from build123d import *

# Parameters (mm, degrees)
F0_W     = 10
F0_H     = 10
F1_DEPTH = 20
F2_DEPTH = 10
F3_R     = 0.5


with BuildPart() as f1:
    # F0 (on Front) → F1 (new body)
    with BuildSketch(Plane.XZ):
        with Locations((-5, 0)):
            Rectangle(F0_W, F0_H)
    extrude(amount=F1_DEPTH)

    # F0 (on Front) → F2 (join)
    with BuildSketch(Plane.XZ):
        with Locations((5, 0)):
            Rectangle(F0_W, F0_H)
        with Locations((-5, 0)):
            Rectangle(F0_W, F0_H)
    extrude(amount=F2_DEPTH)

    # F3
    f3_edges = [f1.edges().sort_by_distance(p)[0] for p in [
        (0, 0, 5),
        (10, -5, 5),
        (5, -10, 5),
        (0, -15, 5),
        (-5, -20, 5),
        (-10, -10, 5),
        (0, 0, -5),
        (-10, -10, -5),
        (-5, -20, -5),
        (0, -15, -5),
        (5, -10, -5),
        (10, -5, -5),
        (10, 0, 0),
        (-10, 0, 0),
        (0, -20, 0),
        (-10, -20, 0),
        (10, -10, 0),
    ]]
    fillet(f3_edges, radius=F3_R)


solid = f1.part
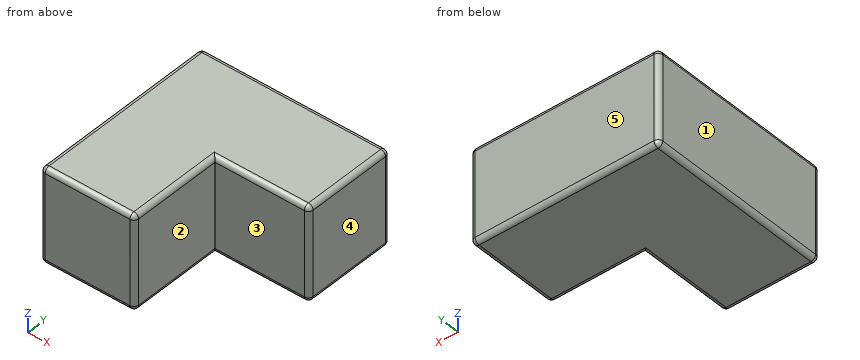
Source: CAD feature listing. Evaluate the final solid. Frame: model axes, mm. Face numbers are marked on the shaded views. A direction names the side the tool comes from. Coordinates: 2 decimals unless noted, no trailing zeros. Order: outer loops, then holes, each group sorted by start corner. A loop starts at its lowest first (then second) coordinate and runs counter-clockwise, first axis right, second up. Notation, with made-up numbers: M 11,25 L 26,25 A27 cw 26,45 Z; hole C 72,-5.75 d9. An arc over 180 degrees is marked long. Write each question's results on one line, items separated by ' | '. Start each with the question number.
Item 1: Cut plane A-A (x = 5.5). Return loops of the section in (y, z).
Item 2: Cut plane B-B (z = -2.5). Return loops of the section in (x, y).
Item 3: First-contact query: pin 1 Ø5 at (x, y) = (3, -14.5) entering from -Z; pin 2 Ø2.5 at (y, z) = (-16, 0) entering from +X; pin 3 Ø2.5 at (x, z) = (3, -1.5) entering from -Y. Flat tips, straight axial feed; report the tip coordinate or a pass-through.
Item 4: Draft query along Y for the marked faces 3, 4 and 5. Return one class per face: pulls with the +Y half, pulls with the -Y half, needs draft (parallel to the pull), parting line crosses it, or undercut.
Item 5: Set-up query: the marked faces 1 and 2. Return all of +Z, -Z, +X, -X, +Y, -Y with unobstructed straight access to the full face (end or side cutting, diameter ignored); none if empty.
Item 6: Line query: probe 1 along X at (y, z) = (-11.5, -0.25). Output: solid intervals per line, ascending.
Checked values:
1) outline: M -10,-4.5 A0.5 ccw -9.5,-5 L -0.5,-5 A0.5 ccw 0,-4.5 L 0,4.5 A0.5 ccw -0.5,5 L -9.5,5 A0.5 ccw -10,4.5 Z
2) outline: M -10,-19.5 A0.5 ccw -9.5,-20 L -0.5,-20 A0.5 ccw 0,-19.5 L 0,-10 L 9.5,-10 A0.5 ccw 10,-9.5 L 10,-0.5 A0.5 ccw 9.5,0 L -9.5,0 A0.5 ccw -10,-0.5 Z
3) pin 1: passes through | pin 2: stops at x = 0 | pin 3: stops at y = -10
4) face 3: pulls with the -Y half | face 4: needs draft | face 5: pulls with the +Y half
5) face 1: +Z, -Z, -X, +Y, -Y | face 2: +Z, -Z, +X, -Y
6) probe 1: x = -10 to 0
